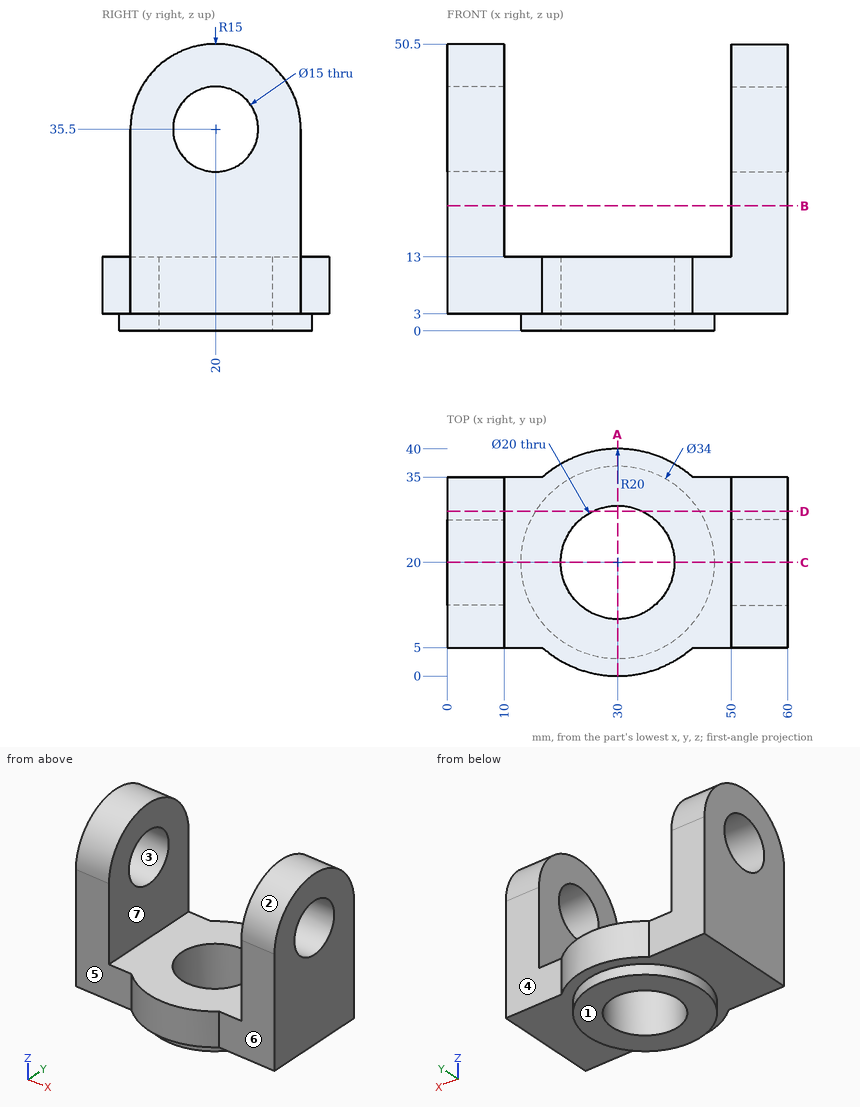
Geometry check sheet. Reference: drawing and pictorial views, mm from the part's lowest x, y, z. A direction names the side the tool comes from. Round coordinates to 2 decimals unless told otherwise and drop trailing zeros. Write each loop counter-clockwise with the first axis right and the second up, starting at its lowest first coordinate (ties: lowest second). Pieces come first, ordered by that corner, then holes.
Item 1: Mould release check, pull along Z, two halves, no side actions. Record for the marked faces 1, 2 and 3: +Z half, -Z half, draft (parallel to the pull), parting line (faces both ways), or undercut.
Determined:
face 1: -Z half
face 2: +Z half
face 3: undercut
Item 2: Section check B-B (z = 22). Record the boundary of the cut face in (x, y), plus the area to 3 significant figures.
Determined:
outline: (0, 5) - (10, 5) - (10, 35) - (0, 35) - close; (50, 5) - (60, 5) - (60, 35) - (50, 35) - close
area: 600 mm2
Item 3: Section check D-D (y = 29). Record the boundary of the cut face in (x, z), plus the area to 3 significant figures.
Determined:
outline: (0, 3) - (15.58, 3) - (15.58, 0) - (25.64, 0) - (25.64, 13) - (10, 13) - (10, 47.5) - (0, 47.5) - close; (34.36, 0) - (44.42, 0) - (44.42, 3) - (60, 3) - (60, 47.5) - (50, 47.5) - (50, 13) - (34.36, 13) - close
area: 1,260 mm2
Item 4: Section check A-A (x = 30). Record the boundary of the cut face in (y, z), plus the area to 3 significant figures.
Determined:
outline: (0, 3) - (3, 3) - (3, 0) - (10, 0) - (10, 13) - (0, 13) - close; (30, 0) - (37, 0) - (37, 3) - (40, 3) - (40, 13) - (30, 13) - close
area: 242 mm2
Item 5: Go/stop test with flat-tipped pins: pin 1 Ø13.5 at (x, z) = (54.5, 13) entering from +Y; pin 2 Ø8.5 at (x, z) = (11.5, 15.5) entering from -Y; pin 3 Ø1 at (x, y) = (25.5, 7) entering from +Z; pin 4 Ø12 at (y, z) = (20, 35.5) entering from -X. Record where each tip stops, or that it passes through.
Determined:
pin 1: stops at y = 35
pin 2: stops at y = 5
pin 3: stops at z = 13
pin 4: passes through
Item 6: Material ranges on line 1 along X through (y, z) = (20, 5); line 2 along Z through (x, y) = (55.75, 20); line 3 along Z through (x, y) = (33.5, 38), recorded low to high.
Determined:
line 1: x = 0 to 20, 40 to 60
line 2: z = 3 to 28, 43 to 50.5
line 3: z = 3 to 13
Item 7: Access from +Z, -Z, +X, -X, +Y, -Y to the whole of each face (thin tool, end or side, straight path). Record for the marked faces 4, 5, 6 and 7.
Determined:
face 4: +Z, -Z, +X, +Y
face 5: +Z, -Z, -X, -Y
face 6: +Z, -Z, +X, -Y
face 7: +Z, +Y, -Y
Item 8: Section check C-C (y = 20). Record the boundary of the cut face in (x, z), plus the area to 3 significant figures.
Determined:
outline: (0, 3) - (13, 3) - (13, 0) - (20, 0) - (20, 13) - (10, 13) - (10, 28) - (0, 28) - close; (0, 43) - (10, 43) - (10, 50.5) - (0, 50.5) - close; (40, 0) - (47, 0) - (47, 3) - (60, 3) - (60, 28) - (50, 28) - (50, 13) - (40, 13) - close; (50, 43) - (60, 43) - (60, 50.5) - (50, 50.5) - close
area: 892 mm2
